Geometry: final body of the model. Coordinates: model frame, mm. Face numbers are marked on the shaded views. Round coordinates to 2 decimals unless told otherwise and drop trailing zeros. Loops run counter-clockwise (first coordinate to the right, second up) from the corner with the lowest first, then second, coordinate; pieces in that order, holes last. Notation, with made-up numbers: M 2,6.5 L 60,6.5 A13 ccw 60,17.5 Z; hole C -3,53 d1. An arc over 180 degrees is marked long. Answer as a JSON object with one key per item and string values.
```python
from build123d import *

# Parameters (mm, degrees)
SKETCH1_R           = 20
SKETCH1_R_2         = 2
BOSS_EXTRUDE1_DEPTH = 16
SKETCH2_R           = 2
CUT_EXTRUDE1_DEPTH  = 33.496153619


with BuildPart() as part:
    # Sketch1 → Boss-Extrude1 (new body)
    with BuildSketch(Plane(origin=(0, 0, 0), x_dir=(1, 0, 0), z_dir=(0, 1, 0))):
        with Locations(Location((0, 0, 0), (0, 0, 270))):
            Circle(SKETCH1_R)
        with Locations(Location((0, 15.5, 0), (0, 0, 270))):
            Circle(SKETCH1_R_2, mode=Mode.SUBTRACT)
        with Locations(Location((15.5, 0, 0), (0, 0, 270))):
            Circle(SKETCH1_R_2, mode=Mode.SUBTRACT)
        with Locations(Location((0, -15.5, 0), (0, 0, 270))):
            Circle(SKETCH1_R_2, mode=Mode.SUBTRACT)
        with Locations(Location((-15.5, 0, 0), (0, 0, 270))):
            Circle(SKETCH1_R_2, mode=Mode.SUBTRACT)
    extrude(amount=BOSS_EXTRUDE1_DEPTH)

    # Sketch2 → Cut-Extrude1 (cut, through all)
    with BuildSketch(Plane(origin=(0, 16, 0), x_dir=(1, 0, 0), z_dir=(0, 1, 0))):
        with Locations(Location((0, 0, 0), (0, 0, 270))):
            Circle(SKETCH2_R)
        with Locations(Location((5.5, 0, 0), (0, 0, 270))):
            Circle(SKETCH2_R)
        with Locations(Location((-5.5, 0, 0), (0, 0, 270))):
            Circle(SKETCH2_R)
    extrude(amount=-CUT_EXTRUDE1_DEPTH, mode=Mode.SUBTRACT)


solid = part.part
```
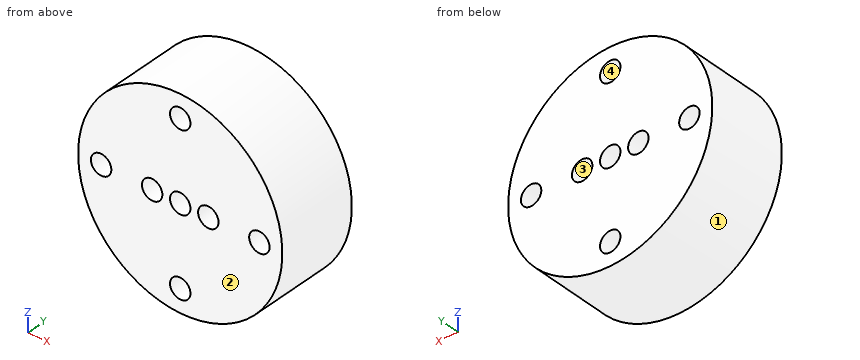
1) Cut plane D-D on x = 15. Return the cut outline in (y, z).
Geometry results:
{"outline": "M 0,-13.23 L 16,-13.23 L 16,-1.94 L 0,-1.94 Z; M 0,1.94 L 16,1.94 L 16,13.23 L 0,13.23 Z"}
2) Line query: probe 1 along X at (y, z) = (11.25, 0); probe 2 along Z at (x, y) = (0.5, 7); probe 3 along X at (y, z) = (5.75, 15.5). Output: solid intervals per line, ascending.
Geometry results:
{"probe 1": "-20 to -17.5, -13.5 to -7.5, -3.5 to -2, 2 to 3.5, 7.5 to 13.5, 17.5 to 20", "probe 2": "-19.99 to -17.44, -13.56 to -1.94, 1.94 to 13.56, 17.44 to 19.99", "probe 3": "-12.64 to -2, 2 to 12.64"}
3) Pull-direction query (Z, two-part tool) for the marked faces 1, 2, 3 and 4; classes: +Z half, -Z half, draft (parallel to the pull), parting line (faces both ways), or undercut.
Geometry results:
{"face 1": "parting line", "face 2": "draft", "face 3": "undercut", "face 4": "undercut"}
4) Cut plane A-A on x = 0. Return the cut outline in (y, z).
Geometry results:
{"outline": "M 0,-20 L 16,-20 L 16,-17.5 L 0,-17.5 Z; M 0,-13.5 L 16,-13.5 L 16,-2 L 0,-2 Z; M 0,2 L 16,2 L 16,13.5 L 0,13.5 Z; M 0,17.5 L 16,17.5 L 16,20 L 0,20 Z"}
5) First-contact query: pin 1 (5 mm diameter, centred on x = -9.5, y = 12.5, fed in from -Z) (3 decimals); pin 2 (3 mm diameter, centred on x = 15.5, z = 0, fed in from -Y); pin 3 (3 mm diameter, centred on x = 13, y = 2, fed in from +Z); pin 4 (8 mm diameter, centred on y = 11.5, z = -8.5, fed in from -X). Flat tips, straight axial feed; report the tip coordinate or a pass-through.
Geometry results:
{"pin 1": "z = -18.735", "pin 2": "through", "pin 3": "z = 16.36", "pin 4": "x = -19.49"}
6) Cut plane C-C on y = 7.5. Return the cut outline in (x, z).
Geometry results:
{"outline": "C 0,0 d40; hole C -15.5,0 d4; hole C -5.5,0 d4; hole C 0,-15.5 d4; hole C 0,0 d4; hole C 0,15.5 d4; hole C 5.5,0 d4; hole C 15.5,0 d4"}
7) Cut plane B-B on z = -15.5. Return the cut outline in (x, y), and give its area (3 significant figures).
Geometry results:
{"outline": "M -12.64,0 L -2,0 L -2,16 L -12.64,16 Z; M 2,0 L 12.64,0 L 12.64,16 L 2,16 Z", "area": "340 mm2"}
